Source: CAD feature listing. Evaluate the final solid. Frame: model axes, mm. A direction names the side the tool comes from. Round coordinates to 2 decimals unless told otherwise and drop trailing zeros. Order: outer loops, then holes, each group sorted by start corner. A loop starts at its lowest first (then second) coordinate and runs counter-clockwise, first axis right, second up. Notation, with made-up numbers: M -8,49 L 32,49 A34 cw 32,88 Z; hole C 22.25,26 d2. An arc over 180 degrees is marked long. Answer as CSV lines item,"result". Start each with the question number.
Item 1: Section query D-D on x = 60.5. Return the cut outline in (y, z), plus the area to 3 significant figures.
Item 2: Section query C-C on y = 14.5. Return the cut outline in (x, z), plus the area to 3 significant figures.
Item 3: Set-up query: faces 1 (the face through (69.55, 23.32, -77.03)), 2 (the face through (1, 19, -79)), 3 (the face through (1, 3, 18)). Return all of +Z, -Z, +X, -X, +Y, -Y with unobstructed straight access to the full face (end or side cutting, diameter ignored); none if empty.
Item 4: Line query: line 1 (Z direction, x = 11.5, y = 25); line 2 (Z direction, x = 0, y = 36.75). Output: solid intervals per line, ascending. Write a range as [from, to].
Item 5: Section query B-B on x = -57. Return the cut outline in (y, z).
Item 6: Pull-direction query (X, two-part tool) for faces 4 (the face through (47, 8.5, -77)), 5 (the face through (0, 43, 0)), 6 (the face through (79, 19, 1)); classes: +X half, -X half, draft (parallel to the pull), parting line (faces both ways), or undercut.
Item 7: First-contact query: P1, Ø8, axis at x = 43.5, z = -8.5, coming from the +Y side; P2, Ø5, axis at x = 25.5, z = -1, coming from the +Y side. Flat tips, straight axial feed; report the tip coordinate or a pass-through.
Item 8: Section query A-A on z = -57. Return the cut outline in (x, y).
Autodesk Inventor part; units mm, degrees
ref_plane "Work Plane1" through (-14, 3, -14) normal (0.6321, 0, -0.7749) x (0, 1, 0)
ref_plane "YZ Plane" through (0, 0, 0) normal (1, 0, 0) x (0, 1, 0)
ref_plane "XZ Plane" through (0, 0, 0) normal (0, 1, 0) x (-1, 0, 0)
sketch "Sketch1" plane through (0, 0, 0) normal (0, 1, 0) x (-1, 0, 0)
  line L0 (-75, 75) -> (75, 75)
  line L1 (75, 75) -> (75, -75)
  line L2 (75, -75) -> (-75, -75)
  line L3 (-75, -75) -> (-75, 75)
  line L4 (-75, 75) -> (75, -75) construction
  line L5 (75, 75) -> (-75, -75) construction
  line L6 (14, 14) -> (-14, 14)
  line L7 (-14, 14) -> (-14, -14)
  line L8 (-14, -14) -> (14, -14)
  line L9 (14, -14) -> (14, 14)
  line L10 (14, 14) -> (-14, -14) construction
  line L11 (-14, 14) -> (14, -14) construction
  circle A0 centre (0, 0) radius 35
  line L12 (-79, -79) -> (79, -79)
  line L13 (79, -79) -> (79, 79)
  line L14 (79, 79) -> (-79, 79)
  line L15 (-79, 79) -> (-79, -79)
  dimension "d0" = 150
  dimension "d1" = 150
  dimension "d2" = 28
  dimension "d3" = 28
  dimension "d4" = 70
  dimension "d7" = 4
extrude "Extrusion2" add sketch "Sketch1" along normal blind 35 contours L15 L14 L13 L12
extrude "Extrusion3" add sketch "Sketch1" along normal blind 3 contours L0 L1 L2 L3 | L9 L8 L7 L6 | A0
sketch "Sketch2" plane through (0, 3, 0) normal (0, 1, 0) x (1, 0, 0)
  line L0 (-14, -14) -> (14, -14)
  line L1 (14, -14) -> (14, 14)
  line L2 (14, 14) -> (-14, 14)
  line L3 (-14, 14) -> (-14, -14)
  line L4 (-14, -14) -> (14, 14) construction
  line L5 (14, -14) -> (-14, 14) construction
  point P0 (0, 0)
  dimension "d12" = 28
  dimension "d13" = 28
extrude "Extrusion4" add sketch "Sketch2" along normal blind 28
sketch "Sketch3" plane through (0, 31, 0) normal (0, 1, 0) x (1, 0, 0)
  circle A0 centre (0, 0) radius 2
  dimension "d16" = 4
extrude "Extrusion5" add sketch "Sketch3" along normal blind 12
sketch "Sketch4" plane through (0, 3, 0) normal (0, 1, 0) x (1, 0, 0)
  line L0 (-65, 72) -> (65, 72)
  line L1 (65, 72) -> (65, -18)
  line L2 (65, -18) -> (24, -18)
  line L3 (24, -18) -> (24, 24)
  line L4 (24, 24) -> (-24, 24)
  line L5 (-24, 24) -> (-24, -18)
  line L6 (-24, -18) -> (-65, -18)
  line L7 (-65, -18) -> (-65, 72)
  line L8 (-75, -75) -> (-75, 75)
  line L9 (75, 75) -> (75, -75)
  line L10 (-75, 75) -> (75, 75)
  line L11 (-14, 14) -> (14, 14)
  line L12 (-14, 14) -> (-14, -14)
  line L13 (14, 14) -> (14, -14)
  line L14 (39, -68) -> (65, -68)
  line L15 (65, -68) -> (65, -28)
  line L16 (65, -28) -> (39, -28)
  line L17 (39, -28) -> (39, -68)
  line L18 (-14, -14) -> (14, -14)
  point P0 (0, 0)
  point P1 (52, -28)
  point P2 (0, -14)
  dimension "d20" = 10
  dimension "d21" = 3
  dimension "d22" = 10
  dimension "d23" = 10
  dimension "d24" = 10
  dimension "d25" = 90
  dimension "d26" = 40
  dimension "d29" = 26
  dimension "d30" = 10
  dimension "d31" = 10
sketch "Sketch5" plane through (0, 31, 0) normal (0, 1, 0) x (1, 0, 0)
  circle A0 centre (0, 0) radius 45
  circle A1 centre (0, 0) radius 2.5714
  dimension "d32" = 90
sketch "Sketch6" plane through (0, 35, 0) normal (0, 1, 0) x (1, 0, 0)
  line L0 (79, 79) -> (-79, 79)
  line L1 (-79, 79) -> (-79, -79)
  line L2 (79, 79) -> (-79, 79)
  line L3 (-79, 79) -> (-79, -79)
  line L4 (-79, -79) -> (79, -79)
  line L5 (79, -79) -> (79, 79)
  point P0 (0, 0)
extrude "Extrusion6" add sketch "Sketch6" along normal blind 3
sketch "Sketch7" plane through (0, 38, 0) normal (0, 1, 0) x (1, 0, 0)
  circle A0 centre (0, 0) radius 2
  circle A1 centre (0, 0) radius 45
  circle A2 centre (0, 0) radius 2.7692
  dimension "d42" = 90
extrude "Extrusion8" cut sketch "Sketch7" against normal blind 2.75 contours A1 | A2
ref_plane "Work Plane1" through (-14, 3, -14) normal (0.6321, 0, -0.7749) x (0, 1, 0)
sketch "Sketch8" plane through (-14, 3, -14) normal (0.6321, 0, -0.7749) x (0, 1, 0)
  circle A0 centre (37.5996, 19.6977) radius 2
  line L0 (32.25, 17.6977) -> (40, 17.6977)
  point P0 (-3, 19.6977)
extrude "Extrusion9" add sketch "Sketch8" along normal blind 40 and the other way blind 2.625
ref_plane "Work Plane2" through (0, 30.5, 0) normal (0, 1, 0) x (1, 0, 0)
sketch "Sketch9" plane through (0, 30.5, 0) normal (0, 1, 0) x (1, 0, 0)
  point P0 (0, 0)
sketch "Sketch10" plane through (79, 0, 79) normal (1, 0, 0) x (0, 0, -1)
  line L0 (8, 7.5) -> (46.5, 7.5)
  line L1 (46.5, 7.5) -> (46.5, 28)
  line L2 (46.5, 28) -> (8, 28)
  line L3 (8, 28) -> (8, 7.5)
  line L4 (0, 38) -> (158, 38)
  line L5 (0, 0) -> (0, 38)
  point P0 (79, 0)
  dimension "d50" = 38.5
  dimension "d51" = 20.5
  dimension "d52" = 10
  dimension "d53" = 8
sketch "Sketch11" plane through (79, 0, -79) normal (0, 0, -1) x (-1, 0, 0)
  line L0 (13, 29) -> (49.5, 29)
  line L1 (50.5, 28) -> (50.5, 9.5)
  line L2 (49.5, 8.5) -> (13, 8.5)
  line L3 (12, 9.5) -> (12, 28)
  circle A0 centre (9.05, 18.75) radius 2.95
  line L4 (6.964, 16.664) -> (12, 11.6281)
  line L5 (6.964, 20.836) -> (12, 25.8719)
  arc A1 (13, 29) -> (12, 28) centre (13, 28) ccw
  arc A2 (12, 9.5) -> (13, 8.5) centre (13, 9.5) ccw
  arc A3 (49.5, 8.5) -> (50.5, 9.5) centre (49.5, 9.5) ccw
  arc A4 (50.5, 28) -> (49.5, 29) centre (49.5, 28) ccw
  line L6 (0, 0) -> (0, 38)
  line L7 (0, 38) -> (158, 38)
  line L8 (55.536, 16.664) -> (50.5, 11.6281)
  circle A5 centre (53.45, 18.75) radius 2.95
  line L9 (55.536, 20.836) -> (50.5, 25.8719)
  point P0 (79, 0)
  point P1 (50.5, 8.5)
  point P2 (50.5, 29)
  point P3 (12, 8.5)
  point P4 (12, 18.75)
  point P5 (50.5, 18.75)
  dimension "d54" = 38.5
  dimension "d55" = 20.5
  dimension "d56" = 5.9
  dimension "d57" = 1
  dimension "d58" = 12
  dimension "d59" = 9
  dimension "d60" = 0
  dimension "d61" = 135
  dimension "d62" = 135
  dimension "d64" = 0
  dimension "d65" = 5.9
  dimension "d66" = 0
  dimension "d67" = 0
  dimension "d68" = 135
  dimension "d69" = 135
extrude "Extrusion10" cut sketch "Sketch11" against normal blind 19.75
properties part number "GPS-Compass-casing"
Results:
1,outline,"M 0,-79 L 8.5,-79 L 8.5,-75 L 3,-75 L 3,75 L 35,75 L 35,-75 L 29,-75 L 29,-79 L 38,-79 L 38,79 L 0,79 Z"
1,area,"1,120 mm^2"
2,outline,"M -79,-79 L 25.63,-79 L 25.63,-75 L -75,-75 L -75,75 L 75,75 L 75,-75 L 69.87,-75 L 69.87,-79 L 79,-79 L 79,79 L -79,79 Z; M -14,-14 L 14,-14 L 14,14 L -14,14 Z"
2,area,"3,070 mm^2"
3,face 1,"-Z"
3,face 2,"-Z, +X, -X, +Y, -Y"
3,face 3,"none"
4,line 1,"[-79, -75], [-14, 14], [75, 79]"
4,line 2,"[-79, -45], [-2, 2], [45, 79]"
5,outline,"M 0,-79 L 38,-79 L 38,79 L 0,79 Z; hole M 3,-75 L 35,-75 L 35,75 L 3,75 Z"
6,face 4,"undercut"
6,face 5,"draft"
6,face 6,"+X half"
7,P1,"y = 38"
7,P2,"y = 35.25"
8,outline,"M -79,0 L 79,0 L 79,38 L -79,38 Z; hole M -75,3 L 75,3 L 75,35 L -75,35 Z"
